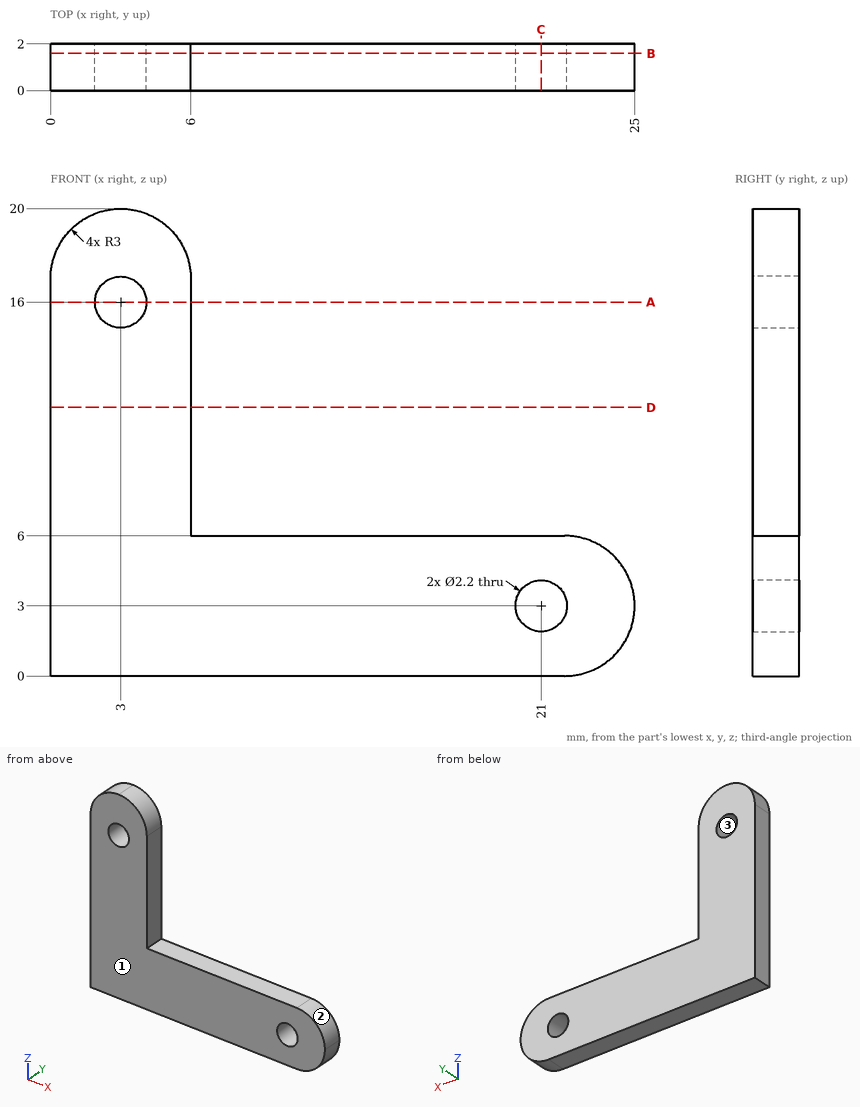
Can you work these out from the drawing? Everything is in mm from the part's minimum corner. Round coordinates to 2 decimals unless told otherwise and drop trailing zeros. Loops run counter-clockwise (first coordinate to the right, second up) from the corner with the lowest first, then second, coordinate; pieces in that order, holes last.
1. We'd pull the mould along Z, two halves only. Please class the marked faces 1, 2 and 3: +Z half, -Z half, draft (parallel to the pull), parting line (faces both ways), or undercut.
Answer list:
face 1: draft
face 2: +Z half
face 3: undercut
2. If we section it at B-B on y = 1.6: Count the separate pieces of the cut face and the enclosed holes in it, plus the area to 3 significant figures.
Answer list:
separate pieces: 1
enclosed holes: 2
area: 219 mm2
3. If we section it at C-C on x = 21: Write out the boundary of the cut face in (y, z), plus the area to 3 significant figures.
Answer list:
outline: (0, 0) - (2, 0) - (2, 1.9) - (0, 1.9) - close; (0, 4.1) - (2, 4.1) - (2, 6) - (0, 6) - close
area: 7.60 mm2
4. If we section it at D-D on z = 11.5: Write out the boundary of the cut face in (x, y).
Answer list:
outline: (0, 0) - (6, 0) - (6, 2) - (0, 2) - close
5. If we section it at A-A on z = 16: Write out the boundary of the cut face in (x, y).
Answer list:
outline: (0, 0) - (1.9, 0) - (1.9, 2) - (0, 2) - close; (4.1, 0) - (6, 0) - (6, 2) - (4.1, 2) - close
6. If I drill on line 1 along X through (y, z) = (0.7, 16); line 2 along Z through (x, y) = (12, 1.6), over which ranges is the centre line in solid material (lowest first)?
Answer list:
line 1: x = 0 to 1.9, 4.1 to 6
line 2: z = 0 to 6
7. For P1, Ø0.6, axis at x = 13.5, y = 1.5, coming from the +Z side, with a flat end and sliding along its axis, tell me the tip position at first contact or that it passes through.
Answer list:
P1: stops at z = 6
